Could you check a few things on this model? Use its own coordinates, in mm. Face numbers are marked on the shaded views. A direction names the side the tool comes from. Give positions to 0.01 mm unless a question says otherwise; leave off trailing zeros. Loops run counter-clockwise (first coordinate to the right, second up) from the corner with the lowest first, then second, coordinate; pieces in that order, holes last. Notation, with made-up numbers: (40, 17.25) -> (57, 17.25) arc R16 ccw to (57, 29.25) -> close; hole circle Ø4 at (-29, 12.5). An arc over 180 degrees is marked (long way). Write each question's results on one line, items separated by ' | '. Start each with the question number.
Q1. If we section it at D-D, the plane y = -17: List the corners of the cut face in (x, z) for me, plus the area to 3 significant figures.
Q2. If we section it at A-A, the plane x = 0: List the corners of the cut face in (y, z) for me.
Q3. Will these pins go through, and if not, where does the flat tip stop? P1, Ø12, axis at x = 3.5, y = -8, coming from the -Z side; P2, Ø11.5, axis at x = -6, y = -12.5, coming from the +Z side; P3, Ø2, axis at y = -30, z = 2, coming from the +X side; P4, Ø2.5, axis at x = 9.5, z = 2.5, coming from the -Y side.
Q4. If I drill on line 1 along Y through (x, z) = (0, 2.55); line 2 along X through (y, z) = (-13, 2.45); line 3 along Y through (x, z) = (0, 1.3), over which ranges is the centre line in solid material (lowest first)?
Q5. If we section it at B-B, the plane y = 12.5: List the corners of the cut face in (x, z) for me.
Q6. Which directions (+Z, -Z, +X, -X, +Y, -Y) give clear straight access to the entire face, cutting with the end or side of a thin tool? Please do the marked faces 4, 5 and 6.
Q7. If we section it at C-C, the plane z = 0.95: List the corners of the cut face in (x, y) for me.
Q8. We'd pull the mould along Y, two halves only. Please class the marked faces 1, 2 and 3: released by +Y, released by -Y, zero draft, split by the parting line, or undercut.
from build123d import *

# Parameters (mm, degrees)
ESQUISSE1_W             = 30
ESQUISSE1_H             = 67
ESQUISSE1_R             = 4
BOSS_EXTRU_1_DEPTH      = 5
ESQUISSE2_W             = 30
ESQUISSE2_H             = 12.5
ENL_V_MAT_EXTRU_1_DEPTH = 5
ESQUISSE3_W             = 5
ESQUISSE3_H             = 5
ENL_V_MAT_EXTRU_2_DEPTH = 38.043892884
BOSS_EXTRU_2_DEPTH      = 5
ENL_V_MAT_EXTRU_3_DEPTH = 40.33509883
ESQUISSE8_W             = 41.113396405
ESQUISSE8_H             = 1
ENL_V_MAT_EXTRU_4_DEPTH = 40.33509883
CONG_1_R                = 10
CONG_2_R                = 10
ESQUISSE9_W             = 24
ESQUISSE9_H             = 13
ENL_V_MAT_EXTRU_5_DEPTH = 3


with BuildPart() as part:
    # Esquisse1 → Boss.-Extru.1 (new body)
    with BuildSketch(Plane.XY):
        Rectangle(ESQUISSE1_W, ESQUISSE1_H)
        with Locations((0, 12.5)):
            Circle(ESQUISSE1_R, mode=Mode.SUBTRACT)
    extrude(amount=BOSS_EXTRU_1_DEPTH)

    # Esquisse2 → Enlèv. mat.-Extru.1 (cut)
    with BuildSketch(Plane.XY.offset(5)):
        with Locations((0, 27.25)):
            Rectangle(ESQUISSE2_W, ESQUISSE2_H)
    extrude(amount=-ENL_V_MAT_EXTRU_1_DEPTH, mode=Mode.SUBTRACT)

    # Esquisse3 → Enlèv. mat.-Extru.2 (cut, through all)
    with BuildSketch(Plane.XY.offset(5)):
        with Locations((-10.5, -31)):
            Rectangle(ESQUISSE3_W, ESQUISSE3_H)
        with Locations((10.5, -31)):
            Rectangle(ESQUISSE3_W, ESQUISSE3_H)
    extrude(amount=-ENL_V_MAT_EXTRU_2_DEPTH, mode=Mode.SUBTRACT)

    # Esquisse5 → Boss.-Extru.2 (add)
    with BuildSketch(Plane.XY.offset(5)):
        Polygon((-15, -19.875), (-20, -33.5), (-15, -33.5), align=None)
        Polygon((15, -19.875), (20, -33.5), (15, -33.5), align=None)
    extrude(amount=-BOSS_EXTRU_2_DEPTH)

    # Esquisse6 → Enlèv. mat.-Extru.3 (cut, through all)
    with BuildSketch(Plane.XY.offset(5)):
        Polygon((-15, 10.78125), (-5, 21), (-15, 21), align=None)
        Polygon((15, 10.78125), (5, 21), (15, 21), align=None)
    extrude(amount=-ENL_V_MAT_EXTRU_3_DEPTH, mode=Mode.SUBTRACT)

    # Esquisse8 → Enlèv. mat.-Extru.4 (cut, through all)
    with BuildSketch(Plane.XY.offset(5)):
        with Locations((0.556698202, -33)):
            Rectangle(ESQUISSE8_W, ESQUISSE8_H)
    extrude(amount=-ENL_V_MAT_EXTRU_4_DEPTH, mode=Mode.SUBTRACT)

    # Congé1
    cong_1_edges = [part.edges().sort_by_distance(p)[0] for p in [
        (-15, 10.78125, 2.5),
        (-5, 21, 2.5),
        (15, 10.78125, 2.5),
        (5, 21, 2.5),
    ]]
    fillet(cong_1_edges, radius=CONG_1_R)

    # Congé2
    cong_2_edges = [part.edges().sort_by_distance(p)[0] for p in [
        (-15, -19.875, 2.5),
        (15, -19.875, 2.5),
    ]]
    fillet(cong_2_edges, radius=CONG_2_R)

    # Esquisse9 → Enlèv. mat.-Extru.5 (cut)
    with BuildSketch(Plane.XY.offset(5)):
        with Locations((0, -4)):
            Rectangle(ESQUISSE9_W, ESQUISSE9_H)
        Polygon((12, -10.5), (-12, -10.5), (-12.5, -10.5), (-12.5, -20.5), (12.5, -20.5), (12.5, -10.5), align=None)
    extrude(amount=-ENL_V_MAT_EXTRU_5_DEPTH, mode=Mode.SUBTRACT)


solid = part.part
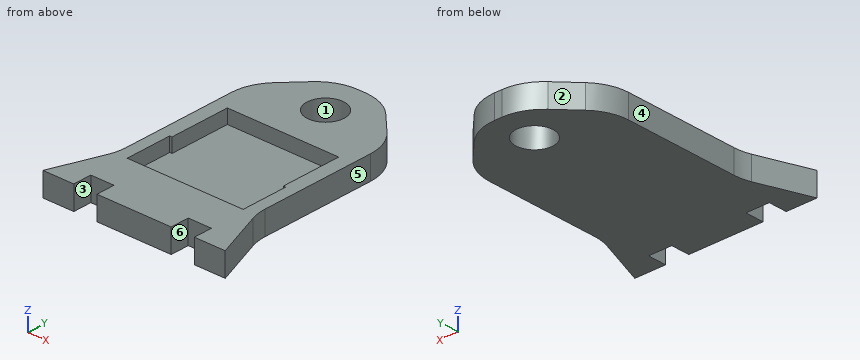
Final values:
1) outline: (-15, 0) -> (15, 0) -> (15, 5) -> (12.5, 5) -> (12.5, 2) -> (-12.5, 2) -> (-12.5, 5) -> (-15, 5) -> close | area: 75.0 mm²
2) outline: (-32.5, 0) -> (8.5, 0) -> (8.5, 5) -> (2.5, 5) -> (2.5, 2) -> (-20.5, 2) -> (-20.5, 5) -> (-32.5, 5) -> close; (16.5, 0) -> (21, 0) -> (21, 5) -> (16.5, 5) -> close
3) P1: stops at z = 0 | P2: stops at z = 2 | P3: stops at x = 19.08 | P4: stops at y = -28.5
4) line 1: y = -32.5 to -20.5, 2.5 to 8.5, 16.5 to 21 | line 2: x = -15 to -12.5, 12.5 to 15 | line 3: y = -32.5 to 8.5, 16.5 to 21
5) outline: (-13.15, 0) -> (-4, 0) -> (-4, 5) -> (-13.15, 5) -> close; (4, 0) -> (13.15, 0) -> (13.15, 5) -> (4, 5) -> close
6) face 4: +Z, -Z, -X, +Y | face 5: +Z, -Z, +X, +Y | face 6: +Z, -Z, -Y
7) outline: (-19.63, -32.5) -> (-13, -32.5) -> (-13, -28.5) -> (-8, -28.5) -> (-8, -32.5) -> (8, -32.5) -> (8, -28.5) -> (13, -28.5) -> (13, -32.5) -> (19.63, -32.5) -> (15.61, -21.54) arc R10 cw to (15, -18.1) -> (15, 6.7) arc R10 ccw to (12.15, 13.7) -> (7.94, 17.99) arc R10 ccw to (0.79, 21) -> (-0.79, 21) arc R10 ccw to (-7.94, 17.99) -> (-12.15, 13.7) arc R10 ccw to (-15, 6.7) -> (-15, -18.1) arc R10 cw to (-15.61, -21.54) -> close; hole circle Ø8 at (0, 12.5)
8) face 1: undercut | face 2: released by +Y | face 3: zero draft
